Read the model definition and answer for the solid it produces. Units are mm, in the model's axes. A direction names the side the tool comes from. Give positions to 0.01 mm unless a question says otherwise; leave off trailing zeros. Order: outer loops, then holes, each group sorted by start corner. A loop starts at its lowest first (then second) coordinate and runs counter-clockwise, first axis right, second up. Notation, with made-up numbers: (85.5, 89) -> (113.5, 89) arc R21 ccw to (113.5, 97) -> close; hole circle Ø8 at (-1, 79.25). An arc over 180 degrees is marked (long way). One line per item, written item: value. Start each with the question number.
from build123d import *

# Parameters (mm, degrees)
SKETCH1_W           = 393.7
SKETCH1_H           = 342.9
BOSS_EXTRUDE1_DEPTH = 355.6
SKETCH2_W           = 50.8
SKETCH2_H           = 44.45
BOSS_EXTRUDE2_DEPTH = 2.54
BOSS_EXTRUDE3_DEPTH = 2.54
SKETCH4_R           = 3.81
CUT_EXTRUDE1_DEPTH  = 2.54
BOSS_EXTRUDE4_DEPTH = 50.8
FILLET1_R           = 6.35
FILLET2_R           = 6.35
SKETCH6_R           = 14.2875
SKETCH6_R_2         = 11.1125
CUT_EXTRUDE2_DEPTH  = 2.54
FILLET3_R           = 19.05
BOSS_EXTRUDE5_DEPTH = 127
FILLET4_R           = 39.116
SKETCH8_W           = 254
SKETCH8_H           = 63.5
CUT_EXTRUDE3_DEPTH  = 25.4
CUT_EXTRUDE4_DEPTH  = 652.703070808
CUT_EXTRUDE5_DEPTH  = 127
BOSS_EXTRUDE6_DEPTH = 127
SKETCH12_W          = 22
SKETCH12_H          = 524.644243645
CUT_EXTRUDE6_DEPTH  = 30
SKETCH13_R          = 63.5
CUT_EXTRUDE7_DEPTH  = 22


with BuildPart() as part:
    # Sketch1 → Boss-Extrude1 (new body)
    with BuildSketch(Plane.XY):
        with Locations((0, 171.45)):
            Rectangle(SKETCH1_W, SKETCH1_H)
    extrude(amount=BOSS_EXTRUDE1_DEPTH)

    # Sketch2 → Boss-Extrude2 (add)
    with BuildSketch(Plane.XY.offset(355.6)):
        with Locations((-133.35, 298.45)):
            Rectangle(SKETCH2_W, SKETCH2_H)
    extrude(amount=BOSS_EXTRUDE2_DEPTH)

    # Sketch3 → Boss-Extrude3 (add)
    with BuildSketch(Plane.XY.offset(355.6)):
        with BuildLine():
            Line((88.9, 307.975), (165.1, 307.975))
            ThreePointArc((165.1, 307.975), (174.625, 298.45), (165.1, 288.925))
            Line((165.1, 288.925), (88.9, 288.925))
            ThreePointArc((88.9, 288.925), (79.375, 298.45), (88.9, 307.975))
        make_face()
    extrude(amount=BOSS_EXTRUDE3_DEPTH)

    # Sketch4 → Cut-Extrude1 (cut)
    with BuildSketch(Plane.XY.offset(358.14)):
        with Locations((92.075, 298.45)):
            Circle(SKETCH4_R)
        with Locations((108.286467636, 298.45)):
            Circle(SKETCH4_R)
        with Locations((124.497935272, 298.45)):
            Circle(SKETCH4_R)
    extrude(amount=-CUT_EXTRUDE1_DEPTH, mode=Mode.SUBTRACT)

    # Sketch5 → Boss-Extrude4 (add)
    with BuildSketch(Plane.XY.offset(355.6)):
        with BuildLine():
            Line((-114.3, 190.5), (114.3, 190.5))
            ThreePointArc((114.3, 190.5), (127, 177.8), (114.3, 165.1))
            Line((114.3, 165.1), (-114.3, 165.1))
            ThreePointArc((-114.3, 165.1), (-127, 177.8), (-114.3, 190.5))
        make_face()
    extrude(amount=BOSS_EXTRUDE4_DEPTH)

    # Fillet1
    fillet1_edges = [part.edges().sort_by_distance(p)[0] for p in [
        (-127, 177.8, 406.4),
        (0, 165.1, 406.4),
        (127, 177.8, 406.4),
        (0, 190.5, 406.4),
    ]]
    fillet(fillet1_edges, radius=FILLET1_R)

    # Fillet2
    fillet2_edges = [part.edges().sort_by_distance(p)[0] for p in [
        (-107.95, 276.225, 356.87),
        (-107.95, 320.675, 356.87),
        (-158.75, 320.675, 356.87),
        (-158.75, 276.225, 356.87),
    ]]
    fillet(fillet2_edges, radius=FILLET2_R)

    # Sketch6 → Cut-Extrude2 (cut)
    # profile 1 of 2: a face of its own
    with BuildSketch(Plane.XY.offset(358.14)):
        with Locations((-133.35, 296.545)):
            Circle(SKETCH6_R)
        with Locations((-133.35, 296.545)):
            Circle(SKETCH6_R_2, mode=Mode.SUBTRACT)
    # profile 2 of 2: a face of its own
    with BuildSketch(Plane.XY.offset(358.14)):
        with BuildLine():
            Line((-134.9375, 296.545), (-134.9375, 315.595))
            ThreePointArc((-134.9375, 315.595), (-133.35, 317.1825), (-131.7625, 315.595))
            Line((-131.7625, 315.595), (-131.7625, 296.545))
            ThreePointArc((-131.7625, 296.545), (-133.35, 294.9575), (-134.9375, 296.545))
        make_face()
    extrude(amount=-CUT_EXTRUDE2_DEPTH, mode=Mode.SUBTRACT)

    # Fillet3
    fillet3_edges = [part.edges().sort_by_distance(p)[0] for p in [
        (196.85, 171.45, 355.6),
        (0, 342.9, 355.6),
        (-196.85, 171.45, 355.6),
        (0, 342.9, 0),
        (196.85, 171.45, 0),
        (0, 0, 0),
        (-196.85, 171.45, 0),
        (0, 0, 355.6),
        (-196.85, 342.9, 177.8),
        (196.85, 342.9, 177.8),
        (196.85, 0, 177.8),
        (-196.85, 0, 177.8),
    ]]
    fillet(fillet3_edges, radius=FILLET3_R)

    # Sketch7 → Boss-Extrude5 (add, symmetric)
    with BuildSketch(Plane(origin=(0, 0, 0), x_dir=(0, 0, -1), z_dir=(1, 0, 0))):
        Polygon((-51.727584486, 342.9), (10.662740116, 469.9), (-31.786520589, 469.9), (-94.17684519, 342.9), align=None)
    extrude(amount=BOSS_EXTRUDE5_DEPTH, both=True)

    # Fillet4
    fillet4_edges = [part.edges().sort_by_distance(p)[0] for p in [
        (-127, 469.9, 10.561890237),
        (127, 469.9, 10.561890237),
    ]]
    fillet(fillet4_edges, radius=FILLET4_R)

    # Sketch8 → Cut-Extrude3 (cut)
    with BuildSketch(Plane(origin=(0, 342.9, 0), x_dir=(1, 0, 0), z_dir=(0, 1, 0))):
        with Locations((0, -125.92684519)):
            Rectangle(SKETCH8_W, SKETCH8_H)
    extrude(amount=-CUT_EXTRUDE3_DEPTH, mode=Mode.SUBTRACT)

    # Sketch9 → Cut-Extrude4 (cut, through all)
    with BuildSketch(Plane(origin=(0, 0, 0), x_dir=(0, 0, -1), z_dir=(1, 0, 0))):
        Polygon((-912.709368589, 769.44705767), (-210.006014515, -1175.153028305), (1122.715383104, 405.705970635), align=None)
    extrude(amount=CUT_EXTRUDE4_DEPTH, mode=Mode.SUBTRACT)

    # Sketch10 → Cut-Extrude5 (cut)
    with BuildSketch(Plane(origin=(0, 0, 0), x_dir=(0, 0, -1), z_dir=(1, 0, 0))):
        Polygon((-94.17684519, 342.9), (-254.864319987, 15.809069962), (-294.760067802, 35.408350722), (-272.360889792, 81.003491082), (-355.6, 121.895736006), (-355.6, 165.1), (-274.492578018, 330.2), (-185.41399178, 286.439040076), (-157.67684519, 342.9), align=None)
    extrude(amount=-CUT_EXTRUDE5_DEPTH, mode=Mode.SUBTRACT)

    # Sketch11 → Boss-Extrude6 (add)
    with BuildSketch(Plane(origin=(0, 0, 0), x_dir=(0, 0, -1), z_dir=(1, 0, 0))):
        Polygon((-94.17684519, 342.9), (-106.65491011, 317.5), (-94.17684519, 317.5), align=None)
    extrude(amount=-BOSS_EXTRUDE6_DEPTH)

    # Sketch12 → Cut-Extrude6 (cut)
    with BuildSketch(Plane(origin=(0, 103.936656142, 211.570550632), x_dir=(1, 0, 0), z_dir=(0, 0.4409287009906531, 0.8975421330738157))):
        with Locations((-11, 164.134434658)):
            Rectangle(SKETCH12_W, SKETCH12_H)
    extrude(amount=-CUT_EXTRUDE6_DEPTH, mode=Mode.SUBTRACT)

    # Sketch13 → Cut-Extrude7 (cut)
    with BuildSketch(Plane(origin=(0, 0, 0), x_dir=(0, 0, -1), z_dir=(1, 0, 0))):
        with Locations((-90.736174491, 196.869487567)):
            Circle(SKETCH13_R)
    extrude(amount=-CUT_EXTRUDE7_DEPTH, mode=Mode.SUBTRACT)


solid = part.part
Item 1: Find section B-B on z = 243. Write down the section's boundary in (x, y).
Item 2: Find the intervals of material crossed by line 1 (Y direction, x = -133, z = 356) (3 decimals); line 2 (Z direction, x = -99, y = 328.5); line 3 (Z direction, x = -132, y = 199.5), in increasing order. Write a range as from..to.
Item 3: Find section A-A on x = -28.5. Write down the section's boundary in (y, z), then the cut area to 3 significant figures.
Item 4: Find section D-D on z = 130. Write down the section's boundary in (x, y).
Item 5: A tool of negligible diameter and unlimited length cuts with its end or side. For faces 5 (the flat face through (-56, 165.1, 378)), 6 (the flat face through (-11.15, 366.13, 49.34)), 7 (the flat face through (-11.15, 86.14, 186.89)), from which of +Z, -Z, +X, -X, +Y, -Y can it reach the whole face along a straight path? Write none if from no direction.
Item 6: Find section C-C on y = 108. Write down the section's boundary in (x, z).
Item 7: For a pull along Z with two mould halves and no side action, classify faces 1 (the cylindrical face through (-87.66, 5.73, 5.43)), 2 (the cylindrical face through (-10.85, 167.13, 34.63)), 3 (the flat face through (-122, 309, 358.14)), 4 (the flat face through (-62.611, 57.887, 283.717)) as +Z half, -Z half, draft (parallel to the pull), parting line (faces both ways), or undercut.
Item 8: Flat-ended cylindrical pins translate along their axes: pin 1 (1 mm diameter, centred on x = -94, z = 289.5, fed in from +Y); pin 2 (2 mm diameter, centred on y = 303, z = 357, fed in from +X); pin 3 (12 mm diameter, centred on x = -106, y = 313, fed in from +Z). Find the tip coordinate at first contact, or state that the pin passes through.
Checks:
1. outline: (-196.85, 19.05) arc R19.05 ccw to (-177.8, 0) -> (0, 0) -> (0, 9.98) -> (-22, 9.98) -> (-22, 39.96) -> (-127, 39.96) -> (-127, 314.73) -> (0, 314.73) -> (0, 342.9) -> (-177.8, 342.9) arc R19.05 ccw to (-196.85, 323.85) -> close
2. line 1: 276.225..282.262, 285.438..294.997, 317.143..320.675
2. line 2: 0.58..101.25, 164.75..271.03, 275.33..355.02
2. line 3: 0..355.6
3. outline: (0, 19.05) arc R19.05 ccw to (19.05, 0) -> (323.85, 0) arc R19.05 ccw to (342.9, 19.05) -> (342.9, 51.73) -> (469.9, -10.66) -> (469.9, 31.79) -> (15.81, 254.86) -> (35.41, 294.76) -> (81, 272.36) -> (121.9, 355.6) -> (19.05, 355.6) arc R19.05 ccw to (0, 336.55) -> close; (165.1, 355.6) -> (330.2, 274.49) -> (286.44, 185.41) -> (342.9, 157.68) -> (342.9, 336.55) arc R19.05 ccw to (323.85, 355.6) -> (190.5, 355.6) -> (190.5, 400.05) arc R6.35 ccw to (184.15, 406.4) -> (171.45, 406.4) arc R6.35 ccw to (165.1, 400.05) -> close
3. area: 87,200 mm2
4. outline: (-196.85, 19.05) arc R19.05 ccw to (-177.8, 0) -> (0, 0) -> (0, 146.96) -> (-22, 146.96) -> (-22, 269.98) -> (-127, 269.98) -> (-127, 342.9) -> (-177.8, 342.9) arc R19.05 ccw to (-196.85, 323.85) -> close
5. face 5: +Z, +X, -X, -Y
5. face 6: +X, +Y
5. face 7: +X
6. outline: (-196.85, 19.05) arc R19.05 ccw to (-177.8, 0) -> (0, 0) -> (0, 176.15) -> (-22, 176.15) -> (-22, 209.57) -> (-127, 209.57) -> (-127, 327.31) -> (0, 327.31) -> (0, 355.6) -> (-177.8, 355.6) arc R19.05 ccw to (-196.85, 336.55) -> close
7. face 1: -Z half
7. face 2: undercut
7. face 3: +Z half
7. face 4: undercut
8. pin 1: y = 342.9
8. pin 2: x = -107.95
8. pin 3: z = 358.14
